```python
from build123d import *

# Parameters (mm, degrees)
SKETCH2_W           = 77
SKETCH2_H           = 40
SKETCH2_W_2         = 3
BOSS_EXTRUDE1_DEPTH = 3
SKETCH2_3_W         = 3
SKETCH2_3_H         = 40
BOSS_EXTRUDE2_DEPTH = 60
FILLET1_R           = 3
SKETCH3_R           = 2
SKETCH3_R_2         = 3.5
CUT_EXTRUDE1_DEPTH  = 81
SKETCH7_R           = 3
CUT_EXTRUDE2_DEPTH  = 64


with BuildPart() as part:
    # Sketch2 → Boss-Extrude1 (new body)
    with BuildSketch(Plane(origin=(0, 0, 0), x_dir=(1, 0, 0), z_dir=(0, 1, 0))):
        with Locations((38.5, 20)):
            Rectangle(SKETCH2_W, SKETCH2_H)
        with Locations((78.5, 20)):
            Rectangle(SKETCH2_W_2, SKETCH2_H)
    extrude(amount=-BOSS_EXTRUDE1_DEPTH)

    # Sketch2_3 → Boss-Extrude2 (add)
    with BuildSketch(Plane(origin=(0, 0, 0), x_dir=(1, 0, 0), z_dir=(0, 1, 0))):
        with Locations((78.5, 20)):
            Rectangle(SKETCH2_3_W, SKETCH2_3_H)
    extrude(amount=BOSS_EXTRUDE2_DEPTH)

    # Fillet1
    fillet1_edges = [part.edges().sort_by_distance(p)[0] for p in [
        (80, -3, -20),
        (77, 0, -20),
    ]]
    fillet(fillet1_edges, radius=FILLET1_R)

    # Sketch3 → Cut-Extrude1 (cut, through all)
    with BuildSketch(Plane(origin=(80, 0, 0), x_dir=(0, 0, -1), z_dir=(1, 0, 0))):
        with BuildLine():
            ThreePointArc((0, 40), (5.857864376, 54.142135624), (20, 60))
            Line((20, 60), (0, 60))
            Line((0, 60), (0, 40))
        make_face()
        with BuildLine():
            Line((40, 60), (20, 60))
            ThreePointArc((20, 60), (34.142135624, 54.142135624), (40, 40))
            Line((40, 40), (40, 60))
        make_face()
        with Locations((20, 50)):
            Circle(SKETCH3_R)
        with Locations((20, 35)):
            Circle(SKETCH3_R)
        with Locations((10, 20)):
            Circle(SKETCH3_R_2)
        with Locations((30, 20)):
            Circle(SKETCH3_R_2)
    extrude(amount=-CUT_EXTRUDE1_DEPTH, mode=Mode.SUBTRACT)

    # Sketch7 → Cut-Extrude2 (cut, through all)
    with BuildSketch(Plane.XZ.offset(3)):
        with Locations((60, -20)):
            Circle(SKETCH7_R)
        with Locations((20, -20)):
            Circle(SKETCH7_R)
    extrude(amount=-CUT_EXTRUDE2_DEPTH, mode=Mode.SUBTRACT)


solid = part.part
```
Build history of the part. All positions in model axes, mm. A direction names the side the tool comes from. Round coordinates to 2 decimals unless told otherwise and drop trailing zeros. Write each loop counter-clockwise with the first axis right and the second up, starting at its lowest first coordinate (ties: lowest second). Pieces come first, ordered by that corner, then holes.
1) Band-saw the part on C-C, the plane z = -30. List the corners of the cut face in (x, y), and give its area (3 significant figures).
2) Mould opens along X. For faces 3 (the cylindrical face through (57, -2, -20)), 4 (the flat face through (52, -1, 0)), 5 (the cylindrical face through (17.6, -1.5, -21.8)), 6 (the flat face through (80, 30, -20)) say: +X half, -X half, draft (parallel to the pull), parting line (faces both ways), or undercut.
3) Band-saw the part on A-A, the plane y = 20. List the corners of the cut face in (x, z), and give its area (3 significant figures).
4) 3-axis set-ups, long thin cutter, end or side, ignore diameter. For faces 1 (the cylindrical face through (79.14, -2.1, -20.28)), 2 (the flat face through (36, 0, -20)): which of +Z, -Z, +X, -X, +Y, -Y reach the whole face in a straight line?
5) Drill centre lines: probe 1 along Z at (x, y) = (20, -1.65); probe 2 along Y at (x, z) = (78, -20); probe 3 along Y at (x, z) = (78.7, -20). Where is each one in solid material? Low to high.
6) Band-saw the part on D-D, the plane y = 35. List the corners of the cut face in (x, z).
7) Pin check, flat tip, straight feed: pin 1 (1.5 mm diameter, centred on x = 36.5, z = -28.5, fed in from +Y). Stop position of the tip, or through.
8) Band-saw the part on B-B, the plane x = 20. List the corners of the cut face in (y, z).
Ans:
1. outline: (0, -3) - (77, -3) arc R3 ccw to (80, 0) - (80, 16.5) - (77, 16.5) - (77, 3) arc R3 cw to (74, 0) - (0, 0) - close; (77, 23.5) - (80, 23.5) - (80, 57.32) - (77, 57.32) - close
1. area: 391 mm2
2. face 3: undercut
2. face 4: draft
2. face 5: undercut
2. face 6: +X half
3. outline: (77, -40) - (80, -40) - (80, -33.5) - (77, -33.5) - close; (77, -26.5) - (80, -26.5) - (80, -13.5) - (77, -13.5) - close; (77, -6.5) - (80, -6.5) - (80, 0) - (77, 0) - close
3. area: 78.0 mm2
4. face 1: +Z, -Z, +X, -Y
4. face 2: +Z, -Z, -X, +Y
5. probe 1: z = -40 to -23, -17 to 0
5. probe 2: y = -2.83 to 33, 37 to 48, 52 to 60
5. probe 3: y = -2.47 to 33, 37 to 48, 52 to 60
6. outline: (77, -40) - (80, -40) - (80, -22) - (77, -22) - close; (77, -18) - (80, -18) - (80, 0) - (77, 0) - close
7. pin 1: stops at y = 0
8. outline: (-3, -40) - (0, -40) - (0, -23) - (-3, -23) - close; (-3, -17) - (0, -17) - (0, 0) - (-3, 0) - close
